The listing builds one solid part. Answer for the finished solid, in the listing's coordinates (mm). A direction names the side the tool comes from. Coordinates: 2 decimals unless noted, no trailing zeros. Order: outer loops, then holes, each group sorted by start corner. A loop starts at its lowest first (then second) coordinate and runs counter-clockwise, first axis right, second up. Notation, with made-up numbers: (-19.5, 79) - (37.5, 79) arc R15 ccw to (37.5, 97) - close; hole circle Ø11 at (-16.5, 46). An arc over 180 degrees is marked (long way). Use a Markdown table: item, result. Add a question column.
Item 1: The part is cut by section B-B, the plane z = 0. Give the vertices of the cut face in (x, y).
Item 2: Find the intervals of material crossed by line 1 along Y through (x, z) = (4.5, -4.5); line 2 along Z through (x, y) = (-4, 139.5); line 3 along Z through (x, y) = (2.25, -11.5), in increasing order.
Item 3: For faces 1 (the cylindrical face through (-6, -10, 0)), 2 (the cylindrical face through (-6, 146, 0)), 3 (the flat face through (0, 67, 7.5)), determine the directions among +Z, -Z, +X, -X, +Y, -Y from which every point of the face is accessible in a straight line to the end or side of a thin tool.
Item 4: The part is cut by section A-A, the plane x = 0. Give the vertices of the cut face in (y, z), then the cut area to 3 significant figures.
from build123d import *

# Parameters (mm, degrees)
SKETCH_1_W      = 15
SKETCH_1_H      = 15
EXTRUDE_1_DEPTH = 136
SKETCH_2_R      = 6
EXTRUDE_2_DEPTH = 20
SKETCH_3_R      = 6
EXTRUDE_3_DEPTH = 20


with BuildPart() as part:
    # 草图1 → 凸台-拉伸1 (new body)
    with BuildSketch(Plane(origin=(0, 0, 0), x_dir=(1, 0, 0), z_dir=(0, 1, 0))):
        Rectangle(SKETCH_1_W, SKETCH_1_H)
    extrude(amount=EXTRUDE_1_DEPTH)

    # 草图2 → 凸台-拉伸2 (add)
    with BuildSketch(Plane(origin=(0, 136, 0), x_dir=(1, 0, 0), z_dir=(0, 1, 0))):
        Circle(SKETCH_2_R)
    extrude(amount=EXTRUDE_2_DEPTH)

    # 草图3 → 凸台-拉伸3 (add)
    with BuildSketch(Plane.XZ):
        Circle(SKETCH_3_R)
    extrude(amount=EXTRUDE_3_DEPTH)


solid = part.part
Solution:
| question | item | result |
|---|---|---|
| 1 | outline | (-7.5, 0) - (-6, 0) - (-6, -20) - (6, -20) - (6, 0) - (7.5, 0) - (7.5, 136) - (6, 136) - (6, 156) - (-6, 156) - (-6, 136) - (-7.5, 136) - close |
| 2 | line 1 | y = 0 to 136 |
| 2 | line 2 | z = -4.47 to 4.47 |
| 2 | line 3 | z = -5.56 to 5.56 |
| 3 | face 1 | -Y |
| 3 | face 2 | +Y |
| 3 | face 3 | +Z, +X, -X, +Y, -Y |
| 4 | outline | (-20, -6) - (0, -6) - (0, -7.5) - (136, -7.5) - (136, -6) - (156, -6) - (156, 6) - (136, 6) - (136, 7.5) - (0, 7.5) - (0, 6) - (-20, 6) - close |
| 4 | area | 2,520 mm2 |
